Model file for the job. Use its own axes, mm. A direction names the side the tool comes from. Coordinates: 2 decimals unless noted, no trailing zeros. Write each loop counter-clockwise with the first axis right and the second up, starting at its lowest first coordinate (ties: lowest second). Pieces come first, ordered by that corner, then holes. Notation, with made-up numbers: M -23,-2 L -19,-2 A5 ccw -19,5 Z; hole C -31.75,-17.75 d11. An arc over 180 degrees is marked long. One line per question, with ' | ' between items. Start each with the question number.
(1) Two-plate mould, pull along Y, no slides. Class faces 5 (the face through (-29.54, -14.14, 1.27)), 6 (the face through (49.126, 1, 4)), 7 (the face through (-21, -33.56, 14)), 8 (the face through (6.94, 14.43, 1.27)): +Y half, -Y half, draft (parallel to the pull), parting line (faces both ways), or undercut.
(2) Cut at A-A (y = 32). Write the cut outline in (x, z), plus the area to 3 significant figures.
(3) Cut at D-D (z = 27.95). Count the separate pieces of the cut face and the enclosed holes in it, plus the area to 3 significant figures.
(4) Cut at B-B (z = 4). Write the cut outline in (x, y).
(5) Cut at C-C (x = -8). Write the cut outline in (y, z), plus the area to 3 significant figures.
(6) Tool access for faces 1 (the face through (26.535, 16, 1)), 2 (the face through (38.901, -4, 5)), 3 (the face through (-24, 33.189, 1)), 4 (the face through (44.5, 0.093, 4.8)): list every direction of +Z, -Z, +X, -X, +Y, -Y with a clear straight run to the whole face (end or side of a thin tool).
(7) Flat gauge pins, fed straight in: pin 1 Ø10 at (x, y) = (-31, 4) entering from +Z; pin 2 Ø2.5 at (y, z) = (-3, 2) entering from +X; pin 3 Ø1.8 at (x, y) = (-40.5, -32) entering from +Z. Where does each tip first touch, or does it go through?
(8) Wall check: probe 1 along X at (y, z) = (-8, 4); probe 2 along Y at (x, z) = (-29.5, 5); probe 3 along X at (y, z) = (42.5, 31.5). Give the ranges that are in metal, low to high.
from build123d import *
from OCP.BRepAlgoAPI import BRepAlgoAPI_Cut
from OCP.TopTools import TopTools_ListOfShape

# Parameters (mm, degrees)
SKETCH1_R           = 1.75
BOSS_EXTRUDE1_DEPTH = 2.5
CUT_EXTRUDE1_DEPTH  = 72.5
SKETCH3_3_W         = 50
SKETCH3_3_H         = 2.25
BOSS_EXTRUDE2_DEPTH = 30
SKETCH6_R           = 1.375
SKETCH6_W           = 32
SKETCH6_H           = 16.3
CUT_EXTRUDE2_DEPTH  = 105.230334086
SKETCH2_R           = 4.25
BOSS_EXTRUDE4_DEPTH = 27.5
SKETCH7_R           = 3.85
BOSS_EXTRUDE5_DEPTH = 5
BOSS_EXTRUDE6_DEPTH = 5.5
CUT_EXTRUDE3_START  = -2.75
SKETCH10_R          = 1.4
CUT_EXTRUDE3_DEPTH  = 13.30605
SKETCH11_R          = 8.539861485
SKETCH11_R_2        = 11.48003937
SKETCH11_R_3        = 7.272091534
SKETCH11_R_4        = 7.519806812
SKETCH11_R_5        = 6.595679845
SKETCH11_R_6        = 6.427948737
SKETCH11_R_7        = 4.197397556
SKETCH11_R_8        = 3.623122109
SKETCH11_R_9        = 3.210730166
CUT_EXTRUDE4_DEPTH  = 5.5


with BuildPart() as part:
    # Sketch1 → Boss-Extrude1 (new body)
    with BuildSketch(Plane.XY):
        with BuildLine():
            Line((-56.464809788, 28.68976821), (-56.464809788, -36.31023179))
            Line((-56.464809788, -36.31023179), (26.535190212, -36.31023179))
            Line((26.535190212, -36.31023179), (26.535190212, -10.463256981))
            Line((26.535190212, -10.463256981), (49.126360761, -10.463256981))
            Line((49.126360761, -10.463256981), (49.126360761, -7.713256981))
            Line((49.126360761, -7.713256981), (42.816561641, -7.713256981))
            Line((42.816561641, -7.713256981), (42.816561641, 0.0927934))
            Line((42.816561641, 0.0927934), (49.126360761, 0.0927934))
            Line((49.126360761, 0.0927934), (49.126360761, 2.8427934))
            Line((49.126360761, 2.8427934), (26.535190212, 2.8427934))
            Line((26.535190212, 2.8427934), (26.535190212, 28.68976821))
            ThreePointArc((26.535190212, 28.68976821), (7.879441831, 42.792705368), (-14.964809788, 47.799695688))
            Line((-14.964809788, 47.799695688), (-56.464809788, 47.799695688))
            Line((-56.464809788, 47.799695688), (-56.464809788, 28.68976821))
        make_face()
        with Locations((-51.464809788, 23.68976821)):
            Circle(SKETCH1_R, mode=Mode.SUBTRACT)
        with Locations(Location((21.535190212, 23.68976821, 0), (0, 0, 180))):
            Circle(SKETCH1_R, mode=Mode.SUBTRACT)
        with Locations((21.535190212, -31.31023179)):
            Circle(SKETCH1_R, mode=Mode.SUBTRACT)
        with Locations(Location((-51.464809788, -31.31023179, 0), (0, 0, 180))):
            Circle(SKETCH1_R, mode=Mode.SUBTRACT)
    extrude(amount=BOSS_EXTRUDE1_DEPTH)

    # Sketch3 → Cut-Extrude1 (cut)
    with BuildSketch(Plane.XY.offset(2.5)):
        Polygon((-45.464809788, 33.189405095), (0.160752733, 33.189405095), (0.160752733, 25.939405095), (-45.464809788, 25.939405095), (-49.713634909, 25.939405095), (-49.713634909, 33.189405095), align=None)
    extrude(amount=-CUT_EXTRUDE1_DEPTH, mode=Mode.SUBTRACT)

    # Sketch3_3 → Boss-Extrude2 (add)
    with BuildSketch(Plane.XY.offset(2.5)):
        with Locations((-20.464809788, -32.43523179)):
            Rectangle(SKETCH3_3_W, SKETCH3_3_H)
        with Locations((-20.464809788, 41.439405095)):
            Rectangle(SKETCH3_3_W, SKETCH3_3_H)
    extrude(amount=BOSS_EXTRUDE2_DEPTH)

    # Sketch6 → Cut-Extrude2 (cut, through all)
    with BuildSketch(Plane.XZ.offset(33.56023179)):
        with Locations((-40.364809788, 27.95)):
            Circle(SKETCH6_R)
        with Locations((-40.364809788, 20.75)):
            Circle(SKETCH6_R)
        with Locations(Location((-0.564809788, 20.75, 0), (0, 0, 90))):
            Circle(SKETCH6_R)
        with Locations(Location((-0.564809788, 27.95, 0), (0, 0, 90))):
            Circle(SKETCH6_R)
        with Locations((-20.464809788, 24.35)):
            Rectangle(SKETCH6_W, SKETCH6_H)
    extrude(amount=-CUT_EXTRUDE2_DEPTH, mode=Mode.SUBTRACT)

    # Sketch2 → Boss-Extrude4 (add)
    with BuildSketch(Plane.XY.offset(2.5)):
        with Locations(Location((32.668616658, -3.474392223, 0), (0, 0, 180))):
            Circle(SKETCH2_R)
    extrude(amount=BOSS_EXTRUDE4_DEPTH)

    # Sketch7 → Boss-Extrude5 (add)
    with BuildSketch(Plane.XY.offset(30)):
        with Locations((32.668616658, -3.474392223)):
            Circle(SKETCH7_R)
    extrude(amount=BOSS_EXTRUDE5_DEPTH)

    # Sketch8 → Boss-Extrude6 (add)
    with BuildSketch(Plane.XY.offset(2.5)):
        Polygon((49.126360761, 2.8427934), (38.901417253, 2.8427934), (38.901417253, -10.463256981), (49.126360761, -10.463256981), (49.126360761, -7.713256981), (42.816561641, -7.713256981), (42.816561641, 0.0927934), (49.126360761, 0.0927934), align=None)
    extrude(amount=BOSS_EXTRUDE6_DEPTH)


with BuildPart() as cut_extrude3_tool:
    # Sketch10 → Cut-Extrude3 (new body)
    with BuildSketch(Plane.XZ.offset(-0.0927934).offset(CUT_EXTRUDE3_START)):
        with Locations(Location((45.971461201, 4, 0), (0, 0, 270))):
            Circle(SKETCH10_R)
    extrude(amount=CUT_EXTRUDE3_DEPTH)


with BuildPart() as part_1:
    add(part.part)

    # Cut-Extrude3: cut by cut_extrude3_tool, with a tolerance
    cut_extrude3_stock = TopTools_ListOfShape()
    cut_extrude3_stock.Append(part_1.part.wrapped)
    cut_extrude3_tools = TopTools_ListOfShape()
    cut_extrude3_tools.Append(cut_extrude3_tool.part.wrapped)
    cut_extrude3_cut = BRepAlgoAPI_Cut()
    cut_extrude3_cut.SetArguments(cut_extrude3_stock)
    cut_extrude3_cut.SetTools(cut_extrude3_tools)
    cut_extrude3_cut.SetFuzzyValue(0.00001)
    cut_extrude3_cut.Build()
    add(Compound.cast(cut_extrude3_cut.Shape()).solids(), mode=Mode.REPLACE)

    # Sketch11 → Cut-Extrude4 (cut)
    with BuildSketch(Plane.XY.offset(2.5)):
        with Locations((-37.685497527, -16.705468454)):
            Circle(SKETCH11_R)
        with Locations((-21.117750948, 6.238516068)):
            Circle(SKETCH11_R_2)
        with Locations((-9.637711577, -16.705468454)):
            Circle(SKETCH11_R_3)
        with Locations((2.898597996, 8.08771742)):
            Circle(SKETCH11_R_4)
        with Locations((8.040859787, -14.56610874)):
            Circle(SKETCH11_R_5)
        with Locations((-44.818935978, 6.238516068)):
            Circle(SKETCH11_R_6)
        with Locations((10.418404807, 23.017872193)):
            Circle(SKETCH11_R_7)
        with Locations((-24.041815555, -16.705468454)):
            Circle(SKETCH11_R_8)
        with Locations((-51.246884715, -8.165606969)):
            Circle(SKETCH11_R_9)
    extrude(amount=-CUT_EXTRUDE4_DEPTH, mode=Mode.SUBTRACT)


solid = part_1.part
Filled in:
1) face 5: undercut | face 6: draft | face 7: -Y half | face 8: undercut
2) outline: M -56.46,0 L -49.71,0 L -49.71,2.5 L -56.46,2.5 Z; M 0.16,0 L 23.46,0 L 23.46,2.5 L 0.16,2.5 Z | area: 75.1 mm²
3) separate pieces: 9 | enclosed holes: 0 | area: 113 mm²
4) outline: M -45.46,-33.56 L 4.54,-33.56 L 4.54,-31.31 L -45.46,-31.31 Z; M -45.46,40.31 L 4.54,40.31 L 4.54,42.56 L -45.46,42.56 Z; C 32.67,-3.47 d8.5; M 38.9,-10.46 L 44.57,-10.46 L 44.57,-7.71 L 42.82,-7.71 L 42.82,0.09 L 44.57,0.09 L 44.57,2.84 L 38.9,2.84 Z; M 47.37,-10.46 L 49.13,-10.46 L 49.13,-7.71 L 47.37,-7.71 Z; M 47.37,0.09 L 49.13,0.09 L 49.13,2.84 L 47.37,2.84 Z
5) outline: M -36.31,0 L -23.79,0 L -23.79,2.5 L -31.31,2.5 L -31.31,16.2 L -33.56,16.2 L -33.56,2.5 L -36.31,2.5 Z; M -9.62,0 L 25.94,0 L 25.94,2.5 L -9.62,2.5 Z; M 33.19,0 L 47.35,0 L 47.35,2.5 L 42.56,2.5 L 42.56,16.2 L 40.31,16.2 L 40.31,2.5 L 33.19,2.5 Z | area: 217 mm²
6) face 1: +Z, -Z, +X, +Y | face 2: +Z, +Y, -Y | face 3: +Z, -Z | face 4: +Z, -Z, +X
7) pin 1: z = 2.5 | pin 2: x = 42.82 | pin 3: z = 32.5
8) probe 1: 38.9 to 44.57, 47.37 to 49.13 | probe 2: -33.56 to -31.31, 40.31 to 42.56 | probe 3: -45.46 to -36.46, -4.46 to 4.54
